Verification items for the finished model (mm, model axes). A direction names the side the tool comes from. Round coordinates to 2 decimals unless told otherwise and drop trailing zeros. Write each loop counter-clockwise with the first axis right and the second up, starting at its lowest first coordinate (ties: lowest second). Pieces come first, ordered by that corner, then holes. Notation, with made-up numbers: (41.5, 23) - (62.5, 23) arc R34 cw to (62.5, 54) - close; hole circle Ø5 at (42, -19.5). An arc over 180 degrees is marked (long way). Answer as a JSON object with one key per item and string values.
```python
from build123d import *

# Parameters (mm, degrees)
CYLINDER265_R     = 0.5
CYLINDER265_DEPTH = 13.5
FILLET221_R       = 0.25
CYLINDER264_R     = 3
CYLINDER264_DEPTH = 12.8
CYLINDER263_R     = 4
CYLINDER263_DEPTH = 13.8
BOX299_W          = 8
BOX299_H          = 4.5
BOX299_DEPTH      = 13.8
BOX298_W          = 9
BOX298_H          = 9
BOX298_DEPTH      = 3.2


with BuildPart() as fillet221:
    # Cylinder265 → Cylinder265 (new body)
    with BuildSketch(Plane.XY):
        Circle(CYLINDER265_R)
    extrude(amount=CYLINDER265_DEPTH)

    # Fillet221
    fillet221_edges = [fillet221.edges().sort_by_distance(p)[0] for p in [
        (-0.5, 0, 0),
    ]]
    fillet(fillet221_edges, radius=FILLET221_R)


with BuildPart() as fillet221_1:
    # Fillet221 placement: moved
    add(fillet221.part.moved(Location((4.5, 4.5, 0))))


with BuildPart() as cilindro264:
    # Cylinder264 → Cylinder264 (new body)
    with BuildSketch(Plane(origin=(4.5, 4.5, 0), x_dir=(1, 0, 0), z_dir=(0, 0, 1))):
        Circle(CYLINDER264_R)
    extrude(amount=CYLINDER264_DEPTH)


with BuildPart() as cilindro263:
    # Cylinder263 → Cylinder263 (new body)
    with BuildSketch(Plane(origin=(4.5, 4.5, 0), x_dir=(1, 0, 0), z_dir=(0, 0, 1))):
        Circle(CYLINDER263_R)
    extrude(amount=CYLINDER263_DEPTH)


with BuildPart() as cubo284:
    # Box299 → Box299 (new body)
    with BuildSketch(Plane(origin=(0.5, 4.5, 0), x_dir=(1, 0, 0), z_dir=(0, 0, 1))):
        with Locations((4, 2.25)):
            Rectangle(BOX299_W, BOX299_H)
    extrude(amount=BOX299_DEPTH)


with BuildPart() as conector_vcc:
    # Box298 → Box298 (new body)
    with BuildSketch(Plane.XY):
        with Locations((4.5, 4.5)):
            Rectangle(BOX298_W, BOX298_H)
    extrude(amount=BOX298_DEPTH)

    # Fusion202: union Cilindro263, Cubo284
    add(cilindro263.part)
    add(cubo284.part)

    # Cut346: cut Cilindro264
    add(cilindro264.part, mode=Mode.SUBTRACT)

    # Fusion203: union Fillet221
    add(fillet221_1.part)


with BuildPart() as conector_vcc_1:
    # Fusion203 placement: moved
    add(conector_vcc.part.moved(Location((-1, -27, 3))))


solid = conector_vcc_1.part
```
Q1. Gauge pin test, flat ends, axial feed: P1, Ø1.5, axis at y = -24, z = 11.5, coming from the -X side; P2, Ø2, axis at x = 4.5, y = -22, coming from the -Z side; P3, Ø1, axis at x = 5.5, z = 7.5, coming from the -Y side; P4, Ø5, axis at x = 6, z = 12, coming from the -Y side. Record the tip position at first contact, or that the pin passes through.
Geometry check:
{"P1": "stops at x = -0.43", "P2": "stops at z = 3", "P3": "stops at y = -26.21", "P4": "stops at y = -26.5"}
Q2. Material ranges on line 1 along Y through (x, z) = (3.5, 10.75); line 2 along Z through (x, y) = (2.75, -23); line 3 along Z through (x, y) = (2.25, -26.5), recorded low to high. Write a range as [from, to].
Geometry check:
{"line 1": "y = [-26.5, -25.5], [-23, -22], [-19.5, -18]", "line 2": "z = [15.8, 16.8]", "line 3": "z = [3, 6.2]"}
Q3. Release check for a two-part mould opening along X. For faces 1 (the flat face through (8, -23, 5)), 2 (the cylindrical face through (3.435, -22.004, 9.437)), 3 (the flat face through (-1, -23, 5)) record: released by +X, released by -X, zero draft, split by the parting line, or undercut.
Geometry check:
{"face 1": "released by +X", "face 2": "undercut", "face 3": "released by -X"}
Q4. Section check C-C, the plane x = 1.75. Record the cut outline in (y, z).
Geometry check:
{"outline": "(-27, 3) - (-24.94, 3) - (-24.94, 15.8) - (-20.06, 15.8) - (-20.06, 3) - (-18, 3) - (-18, 16.8) - (-26.1, 16.8) - (-26.1, 6.2) - (-27, 6.2) - close"}
Q5. Section check D-D, the plane y = -23.5. Record the cut outline in (x, z).
Geometry check:
{"outline": "(-1, 3) - (0.67, 3) - (0.67, 15.8) - (6.33, 15.8) - (6.33, 3) - (8, 3) - (8, 6.2) - (7.37, 6.2) - (7.37, 16.8) - (-0.37, 16.8) - (-0.37, 6.2) - (-1, 6.2) - close"}
Q6. Section check A-A, the plane z = 5.5. Record the cut outline in (x, y).
Geometry check:
{"outline": "(-1, -27) - (8, -27) - (8, -18) - (-1, -18) - close; circle Ø1 at (3.5, -22.5); hole circle Ø6 at (3.5, -22.5)"}
Q7. Set-up check for faces 4 (the flat face through (3, -27, 5)), 5 (the flat face through (7.5, -20, 11)), 6 (the cylindrical face through (2.85, -25.43, 9.31)), 7 (the flat face through (-0.5, -20, 11)), 8 (the flat face through (1, -26, 6.2)): record each of +Z, -Z, +X, -X, +Y, -Y from which the full face is reachable in a straight line by a thin tool's end or side.
Geometry check:
{"face 4": "+Z, -Z, +X, -X, -Y", "face 5": "+Z, +X, +Y, -Y", "face 6": "-Z", "face 7": "+Z, -X, +Y, -Y", "face 8": "+Z, -Y"}
Q8. Section check B-B, the plane y = -19. Record the cut outline in (x, z), then the cut area to 3 significant figures.
Geometry check:
{"outline": "(-1, 3) - (8, 3) - (8, 6.2) - (7.5, 6.2) - (7.5, 16.8) - (-0.5, 16.8) - (-0.5, 6.2) - (-1, 6.2) - close", "area": "114 mm2"}
